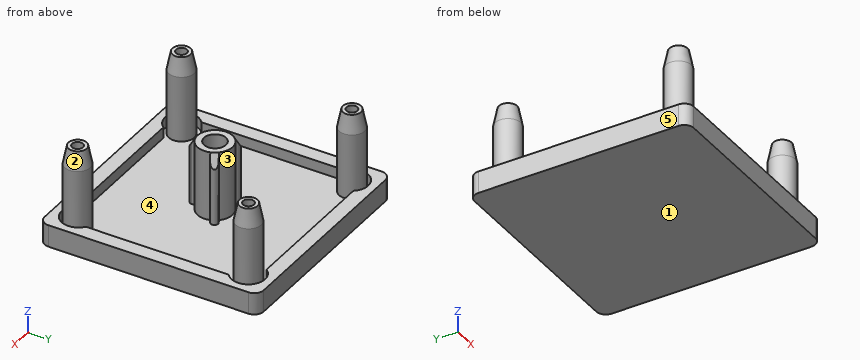
```python
from build123d import *

# Parameters (mm, degrees)
BOSS_EXTRUDE1_DEPTH = 3
CUT_EXTRUDE1_DEPTH  = 1.5
SKETCH8_R           = 6
CUT_EXTRUDE2_DEPTH  = 10


with BuildPart() as part:
    # Sketch1 → Boss-Extrude1 (new body)
    with BuildSketch(Plane.XY):
        with BuildLine():
            Line((-15, 13.7), (-15, -13.7))
            ThreePointArc((-15, -13.7), (-14.619238816, -14.619238816), (-13.7, -15))
            Line((-13.7, -15), (13.7, -15))
            ThreePointArc((13.7, -15), (14.619238816, -14.619238816), (15, -13.7))
            Line((15, -13.7), (15, 13.7))
            ThreePointArc((15, 13.7), (14.619238816, 14.619238816), (13.7, 15))
            Line((13.7, 15), (-13.7, 15))
            ThreePointArc((-13.7, 15), (-14.619238816, 14.619238816), (-15, 13.7))
        make_face()
    extrude(amount=-BOSS_EXTRUDE1_DEPTH)

    # Sketch2 → Cut-Extrude1 (cut)
    with BuildSketch(Plane.XY):
        with BuildLine():
            Line((-13, 9.781260593), (-13, -9.781260593))
            ThreePointArc((-13, -9.781260593), (-13.251345597, -13.251345597), (-9.781260593, -13))
            Line((-9.781260593, -13), (9.781260593, -13))
            ThreePointArc((9.781260593, -13), (13.251345597, -13.251345597), (13, -9.781260593))
            Line((13, -9.781260593), (13, 9.781260593))
            ThreePointArc((13, 9.781260593), (13.251345597, 13.251345597), (9.781260593, 13))
            Line((9.781260593, 13), (-9.781260593, 13))
            ThreePointArc((-9.781260593, 13), (-13.251345597, 13.251345597), (-13, 9.781260593))
        make_face()
    extrude(amount=-CUT_EXTRUDE1_DEPTH, mode=Mode.SUBTRACT)

    # Sketch3 → Revolve1 (revolve)
    with BuildSketch(Plane(origin=(-11.6, 0, 0), x_dir=(0, 0, -1), z_dir=(1, 0, 0)), mode=Mode.PRIVATE) as revolve1_sk:
        Polygon((0, 11.7), (0, 12.45), (-10, 12.45), (-10, 12.95), (-7.5, 13.45), (1.5, 13.45), (1.5, 11.7), align=None)
    revolve(revolve1_sk.sketch.rotate(Axis((-11.6, 11.7, -1.5), (0, 0, 1)), 270), axis=Axis((-11.6, 11.7, -1.5), (0, 0, 1)))

    # Sketch4 → Revolve2 (revolve)
    with BuildSketch(Plane(origin=(11.7, 0, 0), x_dir=(0, 0, -1), z_dir=(1, 0, 0)), mode=Mode.PRIVATE) as revolve2_sk:
        Polygon((0, 11.7), (0, 12.45), (-10, 12.45), (-10, 12.95), (-7.5, 13.45), (1.5, 13.45), (1.5, 11.7), align=None)
    revolve(revolve2_sk.sketch.rotate(Axis((11.7, 11.7, -1.5), (0, 0, 1)), 270), axis=Axis((11.7, 11.7, -1.5), (0, 0, 1)))

    # Sketch5 → Revolve3 (revolve)
    with BuildSketch(Plane(origin=(11.7, 0, 0), x_dir=(0, 0, -1), z_dir=(1, 0, 0)), mode=Mode.PRIVATE) as revolve3_sk:
        Polygon((0, -11.7), (0, -10.95), (-10, -10.95), (-10, -10.45), (-7.5, -9.95), (1.5, -9.95), (1.5, -11.7), align=None)
    revolve(revolve3_sk.sketch.rotate(Axis((11.7, -11.7, -1.5), (0, 0, 1)), 270), axis=Axis((11.7, -11.7, -1.5), (0, 0, 1)))

    # Sketch6 → Revolve4 (revolve)
    with BuildSketch(Plane(origin=(-11.7, 0, 0), x_dir=(0, 0, -1), z_dir=(1, 0, 0)), mode=Mode.PRIVATE) as revolve4_sk:
        Polygon((0, -11.7), (0, -10.95), (-10, -10.95), (-10, -10.45), (-7.5, -9.95), (1.5, -9.95), (1.5, -11.7), align=None)
    revolve(revolve4_sk.sketch.rotate(Axis((-11.7, -11.7, -1.5), (0, 0, 1)), 270), axis=Axis((-11.7, -11.7, -1.5), (0, 0, 1)))

    # Sketch7 → Revolve5 (revolve)
    with BuildSketch(Plane(origin=(0, 0, 0), x_dir=(0, 0, -1), z_dir=(1, 0, 0)), mode=Mode.PRIVATE) as revolve5_sk:
        Polygon((-8, 1.5), (1.5, 1.5), (1.5, 3.4), (-6.267949192, 3.4), (-8, 2.4), align=None)
    revolve(revolve5_sk.sketch.rotate(Axis((0, 0, -10), (0, 0, 1)), 270), axis=Axis((0, 0, -10), (0, 0, 1)))

    # Sketch8 → Cut-Extrude2 (cut)
    with BuildSketch(Plane.XY.offset(-1.5)):
        Circle(SKETCH8_R)
        with BuildLine():
            Line((-2.761473671, 1.016987298), (-2.282855135, 0.740656758))
            ThreePointArc((-2.282855135, 0.740656758), (-2.078460969, -1.2), (-0.5, -2.347338919))
            Line((-0.5, -2.347338919), (-0.5, -2.9))
            ThreePointArc((-0.5, -2.9), (0, -3.4), (0.5, -2.9))
            Line((0.5, -2.9), (0.5, -2.347338919))
            ThreePointArc((0.5, -2.347338919), (2.078460969, -1.2), (2.282855135, 0.740656758))
            Line((2.282855135, 0.740656758), (2.761473671, 1.016987298))
            ThreePointArc((2.761473671, 1.016987298), (2.944486373, 1.7), (2.261473671, 1.883012702))
            Line((2.261473671, 1.883012702), (1.782855135, 1.606682161))
            ThreePointArc((1.782855135, 1.606682161), (0, 2.4), (-1.782855135, 1.606682161))
            Line((-1.782855135, 1.606682161), (-2.261473671, 1.883012702))
            ThreePointArc((-2.261473671, 1.883012702), (-2.944486373, 1.7), (-2.761473671, 1.016987298))
        make_face(mode=Mode.SUBTRACT)
    extrude(amount=CUT_EXTRUDE2_DEPTH, mode=Mode.SUBTRACT)


solid = part.part
```
Geometry check sheet. Reference: the model listing, model coordinates, mm. Face numbers are marked on the shaded views. A direction names the side the tool comes from. Round coordinates to 2 decimals unless told otherwise and drop trailing zeros. Order: outer loops, then holes, each group sorted by start corner. A loop starts at its lowest first (then second) coordinate and runs counter-clockwise, first axis right, second up. Notation, with made-up numbers: M 71.5,33.5 L 75.5,33.5 A31 cw 75.5,72.5 Z; hole C 71.25,39 d9. An arc over 180 degrees is marked long. Write item = value, one per line.
Q1. Depth check by flat-ended pin: pin 1 Ø4 at (y, z) = (9, 2.5) entering from +X; pin 2 Ø1.5 at (x, z) = (-2.5, 4) entering from -Y; pin 3 Ø12 at (x, y) = (1, -2) entering from +Z. Enter the tip coordinate at first touch or a pass-through.
Answer block:
pin_1 = 13.3
pin_2 = -1.64
pin_3 = 8
Q2. Section check B-B (y = 5.75). Enter the section's corners in (x, z).
Answer block:
outline = M -15,-3 L 15,-3 L 15,0 L 13,0 L 13,-1.5 L -13,-1.5 L -13,0 L -15,0 Z
Q3. Set-up check for the marked faces 4 and 5: record each of +Z, -Z, +X, -X, +Y, -Y from which the full face is reachable in a straight line by a thin tool's end or side.
Answer block:
face_4 = +Z
face_5 = +Z, -Z, -X, +Y, -Y
Q4. Section check D-D (x = 0). Enter the section's corners in (y, z).
Answer block:
outline = M -15,-3 L 15,-3 L 15,0 L 13,0 L 13,-1.5 L 2.4,-1.5 L 2.4,8 L 1.5,8 L 1.5,-1.5 L -1.5,-1.5 L -1.5,8 L -2.4,8 L -3.4,6.27 L -3.4,-1.5 L -13,-1.5 L -13,0 L -15,0 Z
Q5. Section check A-A (z = 4.5). Give the number of separate pieces and of enclosed holes in the cut face, plus the area to 3 significant figures.
Answer block:
separate_pieces = 5
enclosed_holes = 5
area = 45.2 mm^2
Q6. Release check for a two-part mould opening along Z. For the marked faces 1, 2 and 3 record: released by +Z, released by -Z, zero draft, split by the parting line, or undercut.
Answer block:
face_1 = released by -Z
face_2 = released by +Z
face_3 = zero draft
Q7. Scan lines: line 1 (Y direction, x = 11.7, z = 4.5); line 2 (X direction, y = 5.5, z = -1); line 3 (Y direction, x = 0, z = 1.5). Record each from-to range of solid material in increasing order.
Answer block:
line_1 = -13.45 to -12.45, -10.95 to -9.95, 9.95 to 10.95, 12.45 to 13.45
line_2 = -15 to -13, 13 to 15
line_3 = -3.4 to -1.5, 1.5 to 2.4
